from build123d import *

# Parameters (mm, degrees)
F0_W     = 100
F0_H     = 30
F1_DEPTH = 10
F2_W     = 50
F2_H     = 30
F3_DEPTH = 30
F4_W     = 100
F4_H     = 130
F4_W_2   = 50
F4_H_2   = 30
F5_DEPTH = 7
F6_W     = 100
F6_H     = 20
F7_DEPTH = 75
F8_R     = 10
F9_DEPTH = 130.001


with BuildPart() as f1:
    # F0 (on Front) → F1 (new body)
    with BuildSketch(Plane.XZ):
        with Locations((16.147754, 1.13822)):
            Rectangle(F0_W, F0_H)
    extrude(amount=F1_DEPTH)

    # F2 (on face) → F3 (join)
    with BuildSketch(Plane.XZ.offset(10)):
        with Locations((16.147754, 1.13822)):
            Rectangle(F2_W, F2_H)
    extrude(amount=F3_DEPTH)

    # F4 (on face) → F5 (join)
    with BuildSketch(Plane.XZ.offset(40)):
        with Locations((16.147754, 1.13822)):
            Rectangle(F4_W, F4_H)
        with Locations((16.147754, 1.13822)):
            Rectangle(F4_W_2, F4_H_2, mode=Mode.SUBTRACT)
        with Locations((16.147754, 1.13822)):
            Rectangle(F4_W_2, F4_H_2)
    extrude(amount=F5_DEPTH)

    # F6 (on face) → F7 (join)
    with BuildSketch(Plane.XZ.offset(47)):
        with Locations((16.147754, -53.86178)):
            Rectangle(F6_W, F6_H)
        with Locations((16.147754, 56.13822)):
            Rectangle(F6_W, F6_H)
    extrude(amount=F7_DEPTH)

    # F8 (on face) → F9 (cut, through all)
    with BuildSketch(Plane.XY.offset(66.13822)):
        with Locations((16.147754, -98.394804)):
            Circle(F8_R)
    extrude(amount=-F9_DEPTH, mode=Mode.SUBTRACT)


solid = f1.part
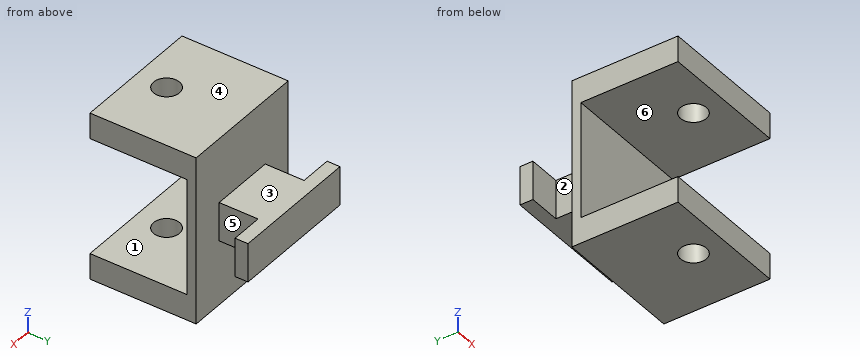
Can you work these out from the model? Positions are in its coordinate system, mm. Face numbers are marked on the shaded views. A direction names the side the tool comes from. Coordinates: 2 decimals unless noted, no trailing zeros. Write each loop counter-clockwise with the first axis right and the second up, starting at its lowest first coordinate (ties: lowest second). Pieces come first, ordered by that corner, then holes.
Q1. For P1, Ø15, axis at y = -21, z = 5, coming from the +X side; P2, Ø4, axis at x = -4, z = -41.5, coming from the -Y side; P3, Ø10, axis at x = -10, z = -46, coming from the +Y side, each with a flat end and sliding along its axis, tell me the tip position at first contact or that it passes through.
Results found:
P1: stops at x = 41.15
P2: stops at y = -47
P3: stops at y = -40
Q2. If we mould it in two halves opening along Z, with no side actions, what happens to the marked faces 4, 5 and 6? For each: +Z half, -Z half, draft (parallel to the pull), parting line (faces both ways), or undercut.
Results found:
face 4: +Z half
face 5: draft
face 6: undercut
Q3. Imagine slicing it at C-C, the plane z = 7.5. List the corners of the cut face in (x, y) for me, plus the area to 3 significant figures.
Results found:
outline: (-33.85, -47) - (66.15, -47) - (66.15, -40) - (41.15, -40) - (41.15, -10) - (66.15, -10) - (66.15, 0) - (-33.85, 0) - (-33.85, -10) - (-8.85, -10) - (-8.85, -40) - (-33.85, -40) - close
area: 3,200 mm2
Q4. Which directions (+Z, -Z, +X, -X, +Y, -Y) give clear straight access to the entire face, cutting with the end or side of a thin tool? Please do the marked faces 1, 2 and 3.
Results found:
face 1: +X, -X, -Y
face 2: +Z, -Z, -X
face 3: +Z, +X, -X, +Y
Q5. Please list where these lines run through material, in increasing order: L1, parallel to Z at x = -2, y = -111; L2, parallel to Y at x = -26, z = 0.5; L3, parallel to Y at x = -21.5, z = 55.
Results found:
L1: z = -63.86 to -43.86, 46.14 to 66.14
L2: y = -47 to -40, -10 to 0
L3: y = -122 to -40
Q6. Imagine slicing it at D-D, the plane z = -51.5. List the corners of the cut face in (x, y) for me.
Results found:
outline: (-33.85, -122) - (66.15, -122) - (66.15, -40) - (-33.85, -40) - close; hole circle Ø20 at (16.15, -98.39)
Q7. Imagine slicing it at B-B, the plane y = -68. List the corners of the cut face in (x, z) for me.
Results found:
outline: (-33.85, -63.86) - (66.15, -63.86) - (66.15, -43.86) - (-33.85, -43.86) - close; (-33.85, 46.14) - (66.15, 46.14) - (66.15, 66.14) - (-33.85, 66.14) - close
Q8. Imagine slicing it at A-A, the plane x = -25.5. List the corners of the cut face in (y, z) for me.
Results found:
outline: (-122, -63.86) - (-40, -63.86) - (-40, 66.14) - (-122, 66.14) - (-122, 46.14) - (-47, 46.14) - (-47, -43.86) - (-122, -43.86) - close; (-10, -13.86) - (0, -13.86) - (0, 16.14) - (-10, 16.14) - close
